Read the model definition and answer for the solid it produces. Units are mm, in the model's axes. Face numbers are marked on the shaded views. Coordinates: 2 decimals unless noted, no trailing zeros. Loops run counter-clockwise (first coordinate to the right, second up) from the corner with the lowest first, then second, coordinate; pieces in that order, holes last.
Q1. Section B-B (x = -14) is taken. Give the vertices of the cut face in (y, z), then the cut area to 3 significant figures.
Q2. Section D-D (z = 28) is taken. Give the vertices of the cut face in (x, y), then the cut area to 3 significant figures.
Q3. Section C-C (z = 15) is taken. Give the vertices of the cut face in (x, y), then the cut area to 3 significant figures.
Q4. The mould has two halves that part along Y. Classify the marked faces 1 and 2: pulls with the +Y half, pulls with the -Y half, needs draft (parallel to the pull), parting line crosses it, or undercut.
Q5. Straight lines are drawn through the part: line 1 (X direction, y = 0, z = 34.5); line 2 (Y direction, x = 0, z = 38.5). For each, find the intervals that lie inside material, in ascending order.
Q6. Section A-A (y = 0) is taken. Give the vertices of the cut face in (x, z).
Q7. Flat-ended cylindrical pins translate along their axes: P1, Ø10, axis at x = -0.5, z = 44.5, coming from the +Y side; P2, Ø3, axis at y = -14.5, z = 17.5, coming from the -X side; P3, Ø1, axis at y = 13, z = 38, coming from the -X side. Find the tip coordinate at first contact, or state that the pin passes through.
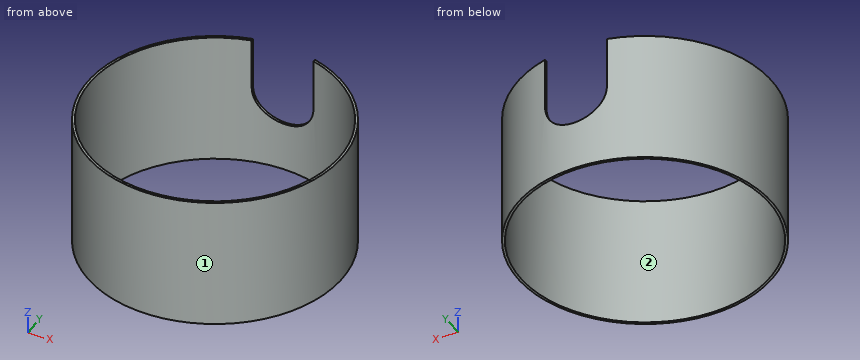
from build123d import *

# Parameters (mm, degrees)
SKETCH1_R           = 50.822
SKETCH1_R_2         = 49.822
BOSS_EXTRUDE1_DEPTH = 53
CUT_EXTRUDE1_DEPTH  = 90.301463415


with BuildPart() as part:
    # Sketch1 → Boss-Extrude1 (new body)
    with BuildSketch(Plane.XY):
        Circle(SKETCH1_R)
        Circle(SKETCH1_R_2, mode=Mode.SUBTRACT)
    extrude(amount=BOSS_EXTRUDE1_DEPTH)

    # Sketch2 → Cut-Extrude1 (cut, through all)
    with BuildSketch(Plane(origin=(0, 0, 0), x_dir=(1, 0, 0), z_dir=(0, 1, 0))):
        with BuildLine():
            Line((-11.666, -32.5), (-11.666, -53))
            Line((-11.666, -53), (13.698, -53))
            Line((13.698, -53), (13.698, -32.5))
            ThreePointArc((13.698, -32.5), (1.016, -19.818), (-11.666, -32.5))
        make_face()
    extrude(amount=CUT_EXTRUDE1_DEPTH, mode=Mode.SUBTRACT)


solid = part.part
Numbers:
1. outline: (-48.86, 0) - (-47.81, 0) - (-47.81, 53) - (-48.86, 53) - close; (47.81, 0) - (48.86, 0) - (48.86, 53) - (47.81, 53) - close
1. area: 110 mm2
2. outline: (-10.84, 48.63) - (-10.84, 49.65) arc R50.82 ccw (long way) to (12.87, 49.16) - (12.87, 48.13) arc R49.82 cw (long way) to start
2. area: 292 mm2
3. outline: circle Ø101.64 at (0, 0); hole circle Ø99.64 at (0, 0)
3. area: 316 mm2
4. face 1: parting line crosses it
4. face 2: undercut
5. line 1: x = -50.82 to -49.82, 49.82 to 50.82
5. line 2: y = -50.82 to -49.82
6. outline: (-50.82, 0) - (-49.82, 0) - (-49.82, 53) - (-50.82, 53) - close; (49.82, 0) - (50.82, 0) - (50.82, 53) - (49.82, 53) - close
7. P1: stops at y = -49.52
7. P2: stops at x = -49.13
7. P3: stops at x = -49.26
